Autodesk Inventor part; units mm, degrees
ref_plane "YZ Plane" through (0, 0, 0) normal (1, 0, 0) x (0, 1, 0)
ref_plane "XZ Plane" through (0, 0, 0) normal (0, 1, 0) x (-1, 0, 0)
ref_plane "XY Plane" through (0, 0, 0) normal (0, 0, 1) x (1, 0, 0)
sketch "Sketch1" plane through (0, 0, 0) normal (0, 0, 1) x (1, 0, 0)
  line L0 (0, 0) -> (24, 0)
  line L1 (24, 0) -> (24, 16)
  line L2 (24, 16) -> (0, 16)
  line L3 (0, 16) -> (0, 0)
  dimension "d0" = 24
  dimension "d1" = 16
extrude "Extrusion1" add sketch "Sketch1" along normal blind 2
fillet "Fillet1" radius 2 4 edges at (0, 16, 1) (0, 0, 1) (24, 0, 1) (24, 16, 1)
sketch "Sketch2" plane through (0, 0, 2) normal (0, 0, 1) x (1, 0, 0)
  line L0 (1.8518, 13.3448) -> (1.8518, 2.0387)
  line L1 (1.8518, 2.0387) -> (3.5541, 2.0387)
  line L2 (3.5541, 2.0387) -> (3.5541, 13.3448)
  line L3 (3.5541, 13.3448) -> (1.8518, 13.3448)
  line L4 (17.1468, 9.3813) -> (17.1468, 3.3599)
  line L5 (17.1468, 3.3599) -> (22.4569, 3.3599)
  line L6 (22.4569, 3.3599) -> (22.4569, 9.3813)
  line L7 (22.4569, 9.3813) -> (17.1468, 9.3813)
  point P0 (0, 0)
extrude "Extrusion2" add sketch "Sketch2" along normal blind 1
properties part number "AmplificadorFInal"
The listing builds one solid part. Answer for the finished solid, in the listing's coordinates (mm). A direction names the side the tool comes from. Give positions to 0.01 mm unless a question says otherwise; leave off trailing zeros. Order: outer loops, then holes, each group sorted by start corner. A loop starts at its lowest first (then second) coordinate and runs counter-clockwise, first axis right, second up. Notation, with made-up numbers: (-15, 49.5) - (-10, 49.5) arc R24 cw to (-10, 65.5) - close; hole circle Ø7 at (-6.5, 19.25). An arc over 180 degrees is marked (long way). Use one line per item in the form item = value.
1) The mould has two halves that part along X. Classify faces 1 (the flat face through (3.554, 7.6, 2.5)), 2 (the flat face through (19.8, 3.36, 2.5)), 3 (the flat face through (24, 8, 1)): released by +X, released by -X, zero draft, split by the parting line, or undercut.
Verdict:
face_1 = undercut
face_2 = zero draft
face_3 = released by +X
2) Find section A-A on y = 5.25. Determine the outline of the cut face in (x, z), and give its area (3 significant figures).
Verdict:
outline = (0, 0) - (24, 0) - (24, 2) - (22.46, 2) - (22.46, 3) - (17.15, 3) - (17.15, 2) - (3.55, 2) - (3.55, 3) - (1.85, 3) - (1.85, 2) - (0, 2) - close
area = 55.0 mm^2
3) Find section D-D on y = 10.25. Determine the outline of the cut face in (x, z).
Verdict:
outline = (0, 0) - (24, 0) - (24, 2) - (3.55, 2) - (3.55, 3) - (1.85, 3) - (1.85, 2) - (0, 2) - close
4) Consider probe 1 along X at (y, z) = (4.5, 2.85); probe 2 along Z at (x, y) = (5.5, 9.75); probe 3 along Y at (x, z) = (2.25, 2.6). Determine where each line is inside the solid, lowest interval first. Write a range as [from, to].
Verdict:
probe_1 = [1.85, 3.55], [17.15, 22.46]
probe_2 = [0, 2]
probe_3 = [2.04, 13.34]
5) Find section C-C on x = 20.25. Determine the outline of the cut face in (y, z).
Verdict:
outline = (0, 0) - (16, 0) - (16, 2) - (9.38, 2) - (9.38, 3) - (3.36, 3) - (3.36, 2) - (0, 2) - close
6) For faces 4 (the flat face through (2.7, 13.345, 2.5)), 5 (the flat face through (1.852, 7.8, 2.5)), 6 (the flat face through (22.457, 6.3, 2.5)), determine the directions among +Z, -Z, +X, -X, +Y, -Y from which every point of the face is accessible in a straight line to the end or side of a thin tool.
Verdict:
face_4 = +Z, +X, -X, +Y
face_5 = +Z, -X, +Y, -Y
face_6 = +Z, +X, +Y, -Y
7) Find section B-B on z = 2.4. Determine the outline of the cut face in (x, y), and give its area (3 significant figures).
Verdict:
outline = (1.85, 2.04) - (3.55, 2.04) - (3.55, 13.34) - (1.85, 13.34) - close; (17.15, 3.36) - (22.46, 3.36) - (22.46, 9.38) - (17.15, 9.38) - close
area = 51.2 mm^2
8) Each of these flat-tipped pins is pushed along its axis until it touches: pin 1 (0.8 mm diameter, centred on y = 7, z = 2.5, fed in from +X); pin 2 (0.8 mm diameter, centred on x = 20.5, z = 2.5, fed in from +Y); pin 3 (5 mm diameter, centred on x = 8, y = 11.5, fed in from +Z). Where does it stop, or does it pass through?
Verdict:
pin_1 = 22.46
pin_2 = 9.38
pin_3 = 2
